Geometry: see drawing. Coordinates: mm, zero at the bounding-box minimum. A direction names the side the tool comes from. Coordinates: 2 decimals unless noted, no trailing zeros. Loops run counter-clockwise (first coordinate to the right, second up) from the corner with the lowest first, then second, coordinate; pieces in that order, holes last. Notation, with made-up numbers: (-28, -39.5) -> (-15, -39.5) arc R27 ccw to (-15, -1.5) -> close; hole circle Ø4 at (10.25, 52.5). An arc over 180 degrees is marked (long way). Answer as a JSON object with one key per item and string values.
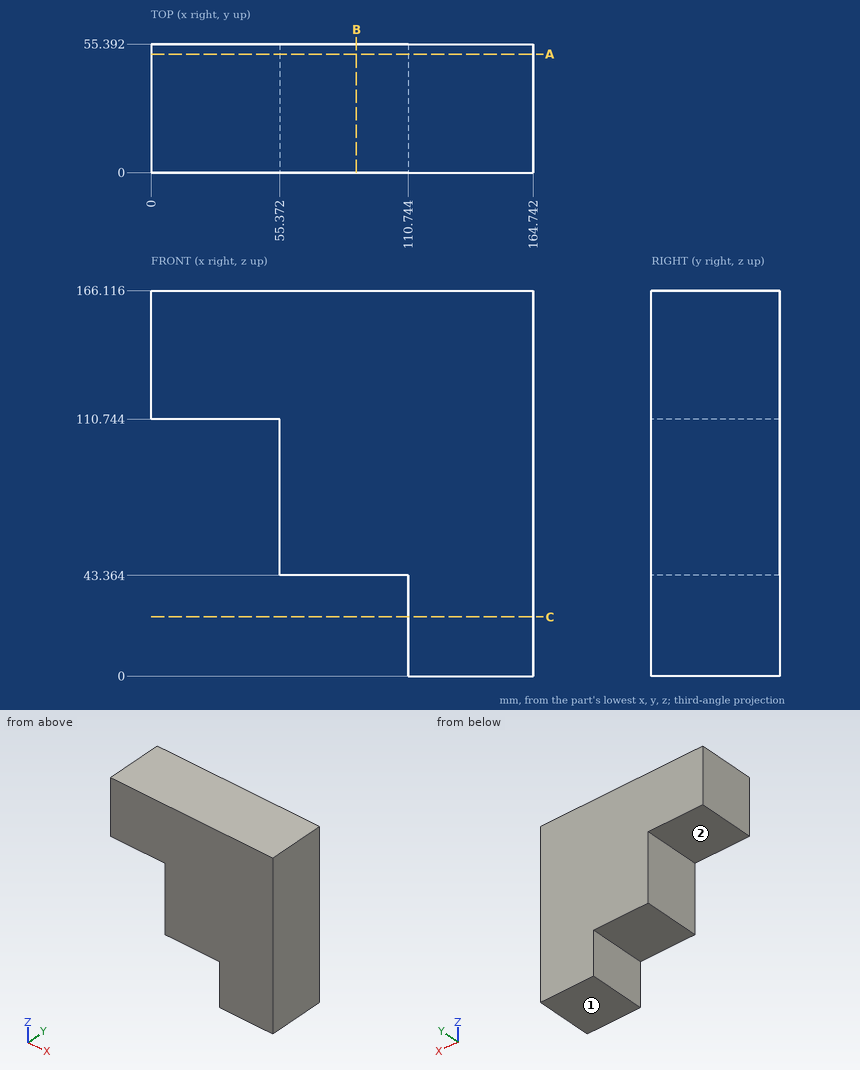
1. Access query for the marked faces 1 and 2. Directions: +Z, -Z, +X, -X, +Y, -Y. A direction counts if a zero-diameter tool reaches every point of the face in a straight line with its end or side. Return the directions, or none.
Reply:
{"face 1": "-Z, +X, -X, +Y, -Y", "face 2": "-Z, -X, +Y, -Y"}
2. Section query B-B (x = 88.5). Return loops of the section in (y, z).
Reply:
{"outline": "(0, 43.36) -> (55.39, 43.36) -> (55.39, 166.12) -> (0, 166.12) -> close"}
3. Section query A-A (y = 51). Return loops of the section in (x, z).
Reply:
{"outline": "(0, 110.74) -> (55.37, 110.74) -> (55.37, 43.36) -> (110.74, 43.36) -> (110.74, 0) -> (164.74, 0) -> (164.74, 166.12) -> (0, 166.12) -> close"}
4. Line query: line 1 along Z through (x, y) = (39, 19); line 2 along X through (y, z) = (44, 71.5); line 3 along Z through (x, y) = (76.5, 27.5). Output: solid intervals per line, ascending.
Reply:
{"line 1": "z = 110.74 to 166.12", "line 2": "x = 55.37 to 164.74", "line 3": "z = 43.36 to 166.12"}
5. Section query C-C (z = 25.5). Return loops of the section in (x, y).
Reply:
{"outline": "(110.74, 0) -> (164.74, 0) -> (164.74, 55.39) -> (110.74, 55.39) -> close"}
6. Pin query (flat end, axial travel): P1, Ø3, axis at x = 110, y = 29, coming from the -Z side; P2, Ø1.5, axis at y = 42, z = 36.5, coming from the -X side. Return the tip coordinate at first contact, or that it passes through.
Reply:
{"P1": "stops at z = 0", "P2": "stops at x = 110.74"}
